Geometry check sheet. Reference: the model listing, model coordinates, mm. A direction names the side the tool comes from. Round coordinates to 2 decimals unless told otherwise and drop trailing zeros. Write each loop counter-clockwise with the first axis right and the second up, starting at its lowest first coordinate (ties: lowest second). Pieces come first, ordered by that corner, then holes. Notation, with made-up numbers: (20, 83) - (54, 83) arc R6 cw to (54, 91) - close; hole circle Ø4 at (-15.5, 78.25). An arc over 180 degrees is marked (long way). Return JSON: item names as keys, results as strings.
```python
from build123d import *

# Parameters (mm, degrees)
F0_R     = 35
F1_DEPTH = 230
F3_R     = 40.5
F3_R_2   = 30.5
F4_DEPTH = 3
F6_R     = 36.6776
F6_R_2   = 30.5
F7_DEPTH = 3
F8_R     = 38.3794
F8_R_2   = 15
F9_DEPTH = 28


# Not quite as in the source:
# - a fillet or chamfer that OpenCascade refuses, or shapes differently, is made with other operations: its cross-section is extruded or revolved along the edge and cut away or added


with BuildPart() as f1:
    # F0 (on Front) → F1 (new body)
    with BuildSketch(Plane.XZ):
        Circle(F0_R)
    extrude(amount=F1_DEPTH)

    # F3 (on offset) + F0 (on Front) → F4 (cut)
    with BuildSketch(Plane(origin=(0, -10, 0), x_dir=(-1, 0, 0), z_dir=(0, 1, 0))):
        Circle(F3_R)
        Circle(F3_R_2, mode=Mode.SUBTRACT)
    with BuildSketch(Plane.XZ):
        Circle(F0_R)
    extrude(amount=-F4_DEPTH, dir=(0, 1, 0), mode=Mode.SUBTRACT)

    # F6 (on offset) → F7 (cut)
    with BuildSketch(Plane(origin=(0, -97, 0), x_dir=(-1, 0, 0), z_dir=(0, 1, 0))):
        Circle(F6_R)
        Circle(F6_R_2, mode=Mode.SUBTRACT)
    extrude(amount=-F7_DEPTH, mode=Mode.SUBTRACT)

    # F8 (on face) → F9 (cut)
    with BuildSketch(Plane.XZ.offset(230)):
        Circle(F8_R)
        Circle(F8_R_2, mode=Mode.SUBTRACT)
    extrude(amount=-F9_DEPTH, mode=Mode.SUBTRACT)

    # F10: fillet of radius 30 on 1 edges, made by hand

    # F10_s1 → F10_t2 (revolve, cut)
    with BuildSketch(Plane.XY):
        with BuildLine():
            ThreePointArc((35, -173.7157287525), (29.4948974278, -191.0362368282), (15, -202))
            Line((15, -202), (35, -202))
            Line((35, -202), (35, -173.7157287525))
        make_face()
    revolve(axis=Axis((0, -202, 0), (0, 1, 0)), mode=Mode.SUBTRACT)


solid = f1.part
```
(1) Material ranges on line 1 along Y through (x, z) = (20.5, 25); line 2 along Z through (x, y) = (-1, -57.5); line 3 along X through (y, z) = (-82, 32.5), recorded low to high. Write a range as [from, to].
Response values:
{"line 1": "y = [-186.09, -100], [-97, -13], [-10, -3]", "line 2": "z = [-34.99, 34.99]", "line 3": "x = [-12.99, 12.99]"}
(2) Gauge pin test, flat ends, axial feed: pin 1 (8 mm diameter, centred on x = 9, y = -33, fed in from -Z); pin 2 (8 mm diameter, centred on x = 17.5, y = -49.5, fed in from +Z); pin 3 (10 mm diameter, centred on x = 8.5, y = -155, fed in from +Z). Record the tip position at first contact, or that the pin passes through.
Response values:
{"pin 1": "stops at z = -34.64", "pin 2": "stops at z = 32.29", "pin 3": "stops at z = 34.82"}
(3) Section check A-A, the plane y = -93. Enter the section's corners in (x, z).
Response values:
{"outline": "circle Ø70 at (0, 0)"}
(4) Section check B-B, the plane y = -215.5. Enter the section's corners in (x, z).
Response values:
{"outline": "circle Ø30 at (0, 0)"}
(5) Access from +Z, -Z, +X, -X, +Y, -Y to the whole of each face (thin tool, end or side, straight path). Record for faces 4 (the face through (11, -97, 29)), 5 (the face through (0, -230, 0)), 6 (the face through (-14.985, -216.196, 0.66)).
Response values:
{"face 4": "none", "face 5": "+Z, -Z, +X, -X, -Y", "face 6": "-Y"}
(6) Release check for a two-part mould opening along Y. For faces 1 (the face through (0, -3, 0)), 2 (the face through (11, -100, 29)), 3 (the face through (-28, -54, -21)) record: pulls with the +Y half, pulls with the -Y half, needs draft (parallel to the pull), parting line crosses it, or undercut.
Response values:
{"face 1": "pulls with the +Y half", "face 2": "undercut", "face 3": "needs draft"}
